The model under review builds one solid part; all positions refer to its coordinate system, in mm. A direction names the side the tool comes from. Round coordinates to 2 decimals unless told otherwise and drop trailing zeros. Write each loop counter-clockwise with the first axis right and the second up, starting at its lowest first coordinate (ties: lowest second). Pieces come first, ordered by that corner, then holes. Notation, with made-up numbers: (-13, -32.75) - (38, -32.75) arc R29 cw to (38, -7.75) - close; hole circle Ø4 at (-6.75, 54). An arc over 180 degrees is marked (long way). Use one line per item in the form item = value.
from build123d import *

# Parameters (mm, degrees)
SKETCH1_W                                      = 53.34
SKETCH1_H                                      = 101.6
PCB_PLATE_DEPTH                                = 3.175
F_4_CLEARANCE_HOLE1_D                          = 3.2639
SKETCH5_W                                      = 56.515
SKETCH5_H                                      = 104.775
SKETCH5_W_2                                    = 53.34
SKETCH5_H_2                                    = 101.6
BORDER_MATERIAL_DEPTH                          = 3.175
SKETCH9_R                                      = 4.365625
BOSS_EXTRUDE3_DEPTH                            = 4.7625
CBORE_FOR_4_SOCKET_HEAD_CAP_SCREW3_D           = 3.2639
CBORE_FOR_4_SOCKET_HEAD_CAP_SCREW3_CBORE_D     = 3.96875
CBORE_FOR_4_SOCKET_HEAD_CAP_SCREW3_CBORE_DEPTH = 4.7625
MATERIAL_REDUCTION_CUT_REACH                   = 61.713
CHAMFER2_SIZE                                  = 0.508


with BuildPart() as part:
    # Sketch1 → PCB Plate (new body)
    with BuildSketch(Plane(origin=(0, 0, 0), x_dir=(1, 0, 0), z_dir=(0, 1, 0))):
        Rectangle(SKETCH1_W, SKETCH1_H)
    extrude(amount=PCB_PLATE_DEPTH)

    # #4 Clearance Hole1 (through all)
    with Locations(Plane(origin=(0, 3.175, 0), x_dir=(1, 0, 0), z_dir=(0, 1, 0))):
        with Locations((-24.13, -36.83), (-24.13, 45.72), (24.13, -35.56), (24.13, 39.37)):
            Hole(F_4_CLEARANCE_HOLE1_D / 2)

    # Sketch5 → Border Material (add)
    with BuildSketch(Plane(origin=(0, 0, 0), x_dir=(1, 0, 0), z_dir=(0, 1, 0))):
        Rectangle(SKETCH5_W, SKETCH5_H)
        Rectangle(SKETCH5_W_2, SKETCH5_H_2, mode=Mode.SUBTRACT)
    extrude(amount=BORDER_MATERIAL_DEPTH)

    # Sketch9 → Boss-Extrude3 (add)
    with BuildSketch(Plane(origin=(0, 3.175, 0), x_dir=(1, 0, 0), z_dir=(0, 1, 0))):
        with Locations(Location((-2.8575, 37.7317, 0), (0, 0, 90))):
            Circle(SKETCH9_R)
        with Locations(Location((-21.11375, 26.6192, 0), (0, 0, 90))):
            Circle(SKETCH9_R)
        with Locations(Location((-2.8575, 15.5067, 0), (0, 0, 90))):
            Circle(SKETCH9_R)
        with Locations(Location((15.39875, 26.6192, 0), (0, 0, 90))):
            Circle(SKETCH9_R)
    extrude(amount=BOSS_EXTRUDE3_DEPTH)

    # CBORE for #4 Socket Head Cap Screw3 (through all)
    with Locations(Plane(origin=(0, 7.9375, 0), x_dir=(1, 0, 0), z_dir=(0, 1, 0))):
        with Locations((-2.8575, 37.7317), (-21.11375, 26.6192), (-2.8575, 15.5067), (15.39875, 26.6192)):
            CounterBoreHole(CBORE_FOR_4_SOCKET_HEAD_CAP_SCREW3_D / 2, CBORE_FOR_4_SOCKET_HEAD_CAP_SCREW3_CBORE_D / 2, CBORE_FOR_4_SOCKET_HEAD_CAP_SCREW3_CBORE_DEPTH)

    # Sketch8 → Material Reduction Cut (cut, up to next)
    with BuildSketch(Plane(origin=(0, 3.175, 0), x_dir=(1, 0, 0), z_dir=(0, 1, 0)), mode=Mode.PRIVATE) as material_reduction_cut_sk1:
        with BuildLine():
            Line((-21.9075, 11.141075), (21.9075, 11.141075))
            Line((21.9075, 11.141075), (21.9075, -27.893708879))
            ThreePointArc((21.9075, -27.893708879), (16.14805, -35.56), (21.9075, -43.226291121))
            Line((21.9075, -43.226291121), (21.9075, -46.0375))
            Line((21.9075, -46.0375), (-21.9075, -46.0375))
            Line((-21.9075, -46.0375), (-21.9075, -44.496291121))
            ThreePointArc((-21.9075, -44.496291121), (-16.14805, -36.83), (-21.9075, -29.163708879))
            Line((-21.9075, -29.163708879), (-21.9075, 11.141075))
        make_face()
    material_reduction_cut_tool1 = extrude(material_reduction_cut_sk1.sketch, amount=-MATERIAL_REDUCTION_CUT_REACH, mode=Mode.PRIVATE) & part.part
    add(material_reduction_cut_tool1.solids().sort_by_distance((0, 3.175, 16.421161))[0], mode=Mode.SUBTRACT)

    # Chamfer2
    chamfer2_edges = [part.edges().sort_by_distance(p)[0] for p in [
        (13.414375, 7.9375, -26.6192),
        (-4.841875, 7.9375, -15.5067),
        (-23.098125, 7.9375, -26.6192),
        (-4.841875, 7.9375, -37.7317),
    ]]
    chamfer(chamfer2_edges, length=CHAMFER2_SIZE)


solid = part.part
(1) Add section A-A on z = -45.72. Write out the cut boundary in (x, y) (1 decimal).
Geometry results:
outline = (-28.3, 0) - (-25.8, 0) - (-25.8, 3.2) - (-28.3, 3.2) - close; (-22.5, 0) - (28.3, 0) - (28.3, 3.2) - (-22.5, 3.2) - close
(2) The part is to be moulded in two halves that separate along X. For faces 4 (the cylindrical face through (-2.5, 1.57, -36.14)), 5 (the flat face through (-1, 7.938, -40)), 6 (the cylindrical face through (-4.17, 5.52, -19.67)), say which applies: +X half, -X half, draft (parallel to the pull), parting line (faces both ways), or undercut.
Geometry results:
face_4 = undercut
face_5 = draft
face_6 = parting line
(3) Add section D-D on y = 6.25. Write out the cut boundary in (x, z), then the cut area to 3 significant figures.
Geometry results:
outline = circle Ø8.73 at (-21.11, -26.62); circle Ø8.73 at (-2.86, -37.73); circle Ø8.73 at (-2.86, -15.51); circle Ø8.73 at (15.4, -26.62); hole circle Ø3.97 at (-21.11, -26.62); hole circle Ø3.97 at (-2.86, -37.73); hole circle Ø3.97 at (-2.86, -15.51); hole circle Ø3.97 at (15.4, -26.62)
area = 190 mm2
(4) Add section C-C on x = -12. Write out the cut boundary in (y, z) (1 decimal), then the cut area to 3 significant figures.
Geometry results:
outline = (0, -52.4) - (3.2, -52.4) - (3.2, -11.1) - (0, -11.1) - close; (0, 46) - (3.2, 46) - (3.2, 52.4) - (0, 52.4) - close
area = 151 mm2
(5) Insertion check: P1, Ø2, axis at x = 24.13, z = 35.56, coming from the +Y side; P2, Ø12, axis at x = 20, z = -16, coming from the +Y side (3 decimals); P3, Ø5, axis at x = -2.86, z = -37.73, coming from the -Y side; P4, Ø1, axis at x = -22, y = 5.5, coming from the -Z side. Each pin has a flat end and moves straight along its axis. Give the tip position at first contact, or say it passes through.
Geometry results:
P1 = through
P2 = 3.175
P3 = 0
P4 = -30.97
(6) Machinability: for faces 1 (the cylindrical face through (16.15, 1.61, 35.42)), 2 (the cylindrical face through (-22.576, 5.332, -27.96)), 3 (the flat face through (0, 2, 52.388)), which of the approach directions +Z, -Z, +X, -X, +Y, -Y give a long, thin tool a straight path to every point of the face, cutting with its end or side? Answer none if there is none.
Geometry results:
face_1 = +Y, -Y
face_2 = +Y
face_3 = +Z, +X, -X, +Y, -Y
(7) Add section B-B on x = 24.13. Write out the cut boundary in (y, z) (1 decimal), then the cut area to 3 significant figures.
Geometry results:
outline = (0, -52.4) - (3.2, -52.4) - (3.2, -41) - (0, -41) - close; (0, -37.7) - (3.2, -37.7) - (3.2, 33.9) - (0, 33.9) - close; (0, 37.2) - (3.2, 37.2) - (3.2, 52.4) - (0, 52.4) - close
area = 312 mm2
(8) To check wall thickness, follow L1, parallel to X at y = 2.5, z = -5; L2, parallel to X at y = 3.5, z = -30.5; L3, parallel to Z at x = -21, y = 6.5. State the ranges of each line that lie inside material, in increasing order.
Geometry results:
L1 = -28.26 to -21.91, 21.91 to 28.26
L2 = -23.11 to -19.11, 13.4 to 17.4
L3 = -30.98 to -28.6, -24.64 to -22.26
